Can you work these out from the model? Positions are in its coordinate system, mm. A direction names the side the tool comes from. Give positions to 0.01 mm unless a question says otherwise; leave off trailing zeros. Order: outer loops, then holes, each group sorted by start corner. A loop starts at its lowest first (then second) coordinate and runs counter-clockwise, first axis right, second up. Notation, with made-up numbers: (-30.75, -32.5) -> (-8.75, -32.5) arc R28 ccw to (-8.75, -11.5) -> close; hole circle Ø9 at (67, -32.75). An arc over 180 degrees is marked (long way). Answer as CSV lines item,"result".
```python
from build123d import *

# Parameters (mm, degrees)
SKETCH1_R                     = 1.575
BOSS_EXTRUDE1_DEPTH           = 2.54
SKETCH2_R                     = 3.175
SKETCH2_R_2                   = 1.575
BOSS_EXTRUDE2_DEPTH           = 0.635
SKETCH3_W                     = 6.35
SKETCH3_H                     = 3
BOSS_EXTRUDE3_DEPTH           = 1
SKETCH4_W                     = 6.35
SKETCH4_H                     = 3
BOSS_EXTRUDE4_DEPTH           = 2
BOSS_EXTRUDE4_DRAFT           = 3
BOSS_EXTRUDE4_PROFILE_2_DEPTH = 2
BOSS_EXTRUDE4_PROFILE_2_DRAFT = 3


with BuildPart() as part:
    # Sketch1 → Boss-Extrude1 (new body)
    with BuildSketch(Plane.XY):
        with BuildLine():
            Line((-184.15, 30.71), (-180.975, 30.71))
            ThreePointArc((-180.975, 30.71), (-180.417860718, 30.58126939), (-179.973667703, 30.221174521))
            Line((-179.973667703, 30.221174521), (-176.593849938, 25.888825479))
            ThreePointArc((-176.593849938, 25.888825479), (-176.149656923, 25.52873061), (-175.592517642, 25.4))
            Line((-175.592517642, 25.4), (-167.307484897, 25.4))
            ThreePointArc((-167.307484897, 25.4), (-166.750344217, 25.528730053), (-166.306150062, 25.888825479))
            Line((-166.306150062, 25.888825479), (-162.926332297, 30.221174521))
            ThreePointArc((-162.926332297, 30.221174521), (-162.482139282, 30.58126939), (-161.925, 30.71))
            Line((-161.925, 30.71), (-155.575, 30.71))
            ThreePointArc((-155.575, 30.71), (-154.676974388, 30.338025612), (-154.305, 29.44))
            Line((-154.305, 29.44), (-154.305, 0))
            Line((-154.305, 0), (-190.5, 0))
            Line((-190.5, 0), (-190.5, 25.4))
            Line((-190.5, 25.4), (-190.5, 29.44))
            ThreePointArc((-190.5, 29.44), (-190.128025612, 30.338025612), (-189.23, 30.71))
            Line((-189.23, 30.71), (-184.15, 30.71))
        make_face()
        with Locations((-184.15, 27.24645)):
            Circle(SKETCH1_R, mode=Mode.SUBTRACT)
    extrude(amount=BOSS_EXTRUDE1_DEPTH)

    # Sketch2 → Boss-Extrude2 (add)
    with BuildSketch(Plane.XY.offset(2.54)):
        with Locations((-184.15, 27.24645)):
            Circle(SKETCH2_R)
        with Locations((-184.15, 27.24645)):
            Circle(SKETCH2_R_2, mode=Mode.SUBTRACT)
    extrude(amount=BOSS_EXTRUDE2_DEPTH)

    # Sketch3 → Boss-Extrude3 (add)
    with BuildSketch(Plane(origin=(0, 0, 0), x_dir=(-1, 0, 0), z_dir=(0, 0, -1))):
        with Locations((184.15, 27.94)):
            Rectangle(SKETCH3_W, SKETCH3_H)
        with Locations((158.75, 27.94)):
            Rectangle(SKETCH3_W, SKETCH3_H)
    extrude(amount=BOSS_EXTRUDE3_DEPTH)


with BuildPart() as boss_extrude4_tool:
    # Sketch4 → Boss-Extrude4 (with draft: the straight prism first)
    with BuildSketch(Plane(origin=(0, 0, -1), x_dir=(-1, 0, 0), z_dir=(0, 0, -1))):
        with Locations((184.15, 27.94)):
            Rectangle(SKETCH4_W, SKETCH4_H)
    extrude(amount=BOSS_EXTRUDE4_DEPTH)
    # Boss-Extrude4: the draft: its side faces are tilted about the plane it starts from
    boss_extrude4_sides = [boss_extrude4_tool.faces().sort_by_distance(p)[0] for p in [
        (-180.975, 27.94, -2),
        (-184.15, 26.44, -2),
        (-187.325, 27.94, -2),
        (-184.15, 29.44, -2),
    ]]
    draft(boss_extrude4_sides, Plane(origin=(0, 0, -1), x_dir=(-1, 0, 0), z_dir=(0, 0, -1)), BOSS_EXTRUDE4_DRAFT)


with BuildPart() as part_1:
    add(part.part)

    # Boss-Extrude4: add boss_extrude4_tool
    add(boss_extrude4_tool.part)


with BuildPart() as boss_extrude4_profile_2_tool:
    # Sketch4 → Boss-Extrude4 profile 2 (with draft: the straight prism first)
    with BuildSketch(Plane(origin=(0, 0, -1), x_dir=(-1, 0, 0), z_dir=(0, 0, -1))):
        with Locations((158.75, 27.94)):
            Rectangle(SKETCH4_W, SKETCH4_H)
    extrude(amount=BOSS_EXTRUDE4_PROFILE_2_DEPTH)
    # Boss-Extrude4 profile 2: the draft: its side faces are tilted about the plane it starts from
    boss_extrude4_profile_2_sides = [boss_extrude4_profile_2_tool.faces().sort_by_distance(p)[0] for p in [
        (-155.575, 27.94, -2),
        (-158.75, 26.44, -2),
        (-161.925, 27.94, -2),
        (-158.75, 29.44, -2),
    ]]
    draft(boss_extrude4_profile_2_sides, Plane(origin=(0, 0, -1), x_dir=(-1, 0, 0), z_dir=(0, 0, -1)), BOSS_EXTRUDE4_PROFILE_2_DRAFT)


with BuildPart() as part_2:
    add(part_1.part)

    # Boss-Extrude4 profile 2: add boss_extrude4_profile_2_tool
    add(boss_extrude4_profile_2_tool.part)

    # Mirror1: part across plane


with BuildPart() as part_3:
    add(part_2.part)
    add(part_2.part.mirror(Plane.ZX))


solid = part_3.part
```
Item 1: For pin 1 (3 mm diameter, centred on x = -185, z = -2, fed in from -Y); pin 2 (12 mm diameter, centred on x = -163, y = -8.5, fed in from -Z); pin 3 (1.9 mm diameter, centred on x = -183.5, y = 28, fed in from +Z) (3 decimals); pin 4 (11 mm diameter, centred on x = -177.5, y = 5.5, fed in from +Z), each with a flat end and sliding along its axis, tell me the tip position at first contact or that it passes through.
Numbers:
pin 1,"stops at y = -29.44"
pin 2,"stops at z = 0"
pin 3,"stops at z = 3.175"
pin 4,"stops at z = 2.54"
Item 2: Imagine slicing it at C-C, the plane y = -1.5. Please give me the cut outline in (x, z) (3 decimals), then the cut area to 3 significant figures.
Numbers:
outline,"(-190.5, 0) -> (-154.305, 0) -> (-154.305, 2.54) -> (-190.5, 2.54) -> close"
area,"91.9 mm²"
Item 3: Imagine slicing it at D-D, the plane x = -173. Please give me the cut outline in (y, z), then the cut area to 3 significant figures.
Numbers:
outline,"(-25.4, 0) -> (25.4, 0) -> (25.4, 2.54) -> (-25.4, 2.54) -> close"
area,"129 mm²"
Item 4: Imagine slicing it at A-A, the plane z = -2. Please give me the cut outline in (x, y).
Numbers:
outline,"(-187.27, -29.39) -> (-181.03, -29.39) -> (-181.03, -26.49) -> (-187.27, -26.49) -> close; (-187.27, 26.49) -> (-181.03, 26.49) -> (-181.03, 29.39) -> (-187.27, 29.39) -> close; (-161.87, -29.39) -> (-155.63, -29.39) -> (-155.63, -26.49) -> (-161.87, -26.49) -> close; (-161.87, 26.49) -> (-155.63, 26.49) -> (-155.63, 29.39) -> (-161.87, 29.39) -> close"
Item 5: Imagine slicing it at B-B, the plane x = -184.15. Give the number of separate pieces and of enclosed holes in the cut face, then the cut area to 3 significant figures.
Numbers:
separate pieces,"3"
enclosed holes,"0"
area,"162 mm²"
Item 6: Please list where these lines run through material, in increasing order: line 1 along Y through (x, z) = (-184.15, 1.1); line 2 along Z through (x, y) = (-171.5, -11.5); line 3 along Y through (x, z) = (-185, -1).
Numbers:
line 1,"y = -30.71 to -28.82, -25.67 to 25.67, 28.82 to 30.71"
line 2,"z = 0 to 2.54"
line 3,"y = -29.44 to -26.44, 26.44 to 29.44"
Item 7: For faces 1 (the flat face through (-164.64, 28.025, 1.252)), 2 (the cylindrical face through (-182.648, -27.72, 1.565)), 3 (the flat face through (-161.873, -27.919, -1.986)), which set-ups out of +Z, -Z, +X, -X, +Y, -Y let a thin tool reach every point of the face, with its end or its side?
Numbers:
face 1,"+Z, -Z, +Y"
face 2,"+Z"
face 3,"-Z, +Y, -Y"
Item 8: We'd pull the mould along Y, two halves only. Please class faces 4 (the cylindrical face through (-182.648, 27.72, 1.565)), 5 (the flat face through (-185, 30.71, 1)), 6 (the flat face through (-155.627, -27.919, -1.986)): released by +Y, released by -Y, zero draft, split by the parting line, or undercut.
Numbers:
face 4,"undercut"
face 5,"released by +Y"
face 6,"zero draft"
